Here's how the part is built. I have some questions about the finished solid (model axes, mm). Face numbers are marked on the shaded views. Round coordinates to 2 decimals unless told otherwise and drop trailing zeros. Loops run counter-clockwise (first coordinate to the right, second up) from the corner with the lowest first, then second, coordinate; pieces in that order, holes last. Notation, with made-up numbers: M 62,-38.75 L 70,-38.75 A21 cw 70,-15.75 Z; hole C 55.25,31.25 d11. An arc over 180 degrees is marked long. Answer as a JSON object with one key per item and string values.
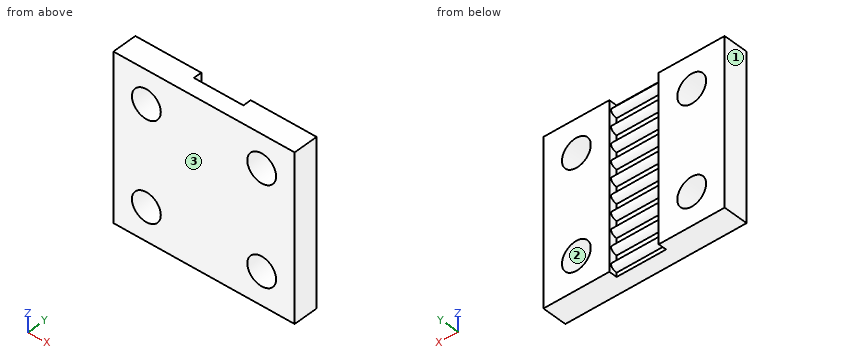
from build123d import *

# Parameters (mm, degrees)
BOSS_EXTRUDE1_DEPTH     = 10
BOSS_EXTRUDE2_START     = -11
SKETCH3_RX              = 0.75
SKETCH3_RY              = 0.5
BOSS_EXTRUDE2_DEPTH     = 14
LPATTERN1_COUNT         = 5
LPATTERN1_PITCH         = 2
LPATTERN1_COL_COUNT     = 6
LPATTERN1_COL_PITCH     = 2
SKETCH4_R               = 1.75
CUT_EXTRUDE2_DEPTH      = 2.0000001
CUT_EXTRUDE2_DEPTH_BACK = 3


with BuildPart() as part:
    # Sketch2 → Boss-Extrude1 (new body, symmetric)
    with BuildSketch(Plane.XY):
        Polygon((-11, 1), (-3, 1), (-3, 0), (3, 0), (3, 1), (11, 1), (11, -2), (-11, -2), align=None)
    extrude(amount=BOSS_EXTRUDE1_DEPTH, both=True)

    # Sketch3 → Boss-Extrude2 (add)
    with BuildSketch(Plane(origin=(0, 0, 0), x_dir=(0, 0, -1), z_dir=(1, 0, 0)).offset(BOSS_EXTRUDE2_START)):
        with Locations(Location((-1, 0), (0, 0, 90))):
            Ellipse(SKETCH3_RX, SKETCH3_RY)
    boss_extrude2 = extrude(amount=BOSS_EXTRUDE2_DEPTH)

    # LPattern1: Boss-Extrude2 ×5
    with Locations(*[(0, 0, i * LPATTERN1_PITCH) for i in range(1, LPATTERN1_COUNT)]):
        add(boss_extrude2)

    # LPattern1 col: Boss-Extrude2 ×6
    with Locations(*[(0, 0, -i * LPATTERN1_COL_PITCH) for i in range(1, LPATTERN1_COL_COUNT)]):
        add(boss_extrude2)

    # Sketch4 → Cut-Extrude2 (cut, two sides)
    with BuildSketch(Plane(origin=(0, 0, 0), x_dir=(1, 0, 0), z_dir=(0, 1, 0))) as cut_extrude2_sk:
        with Locations((-7, 6)):
            Circle(SKETCH4_R)
        with Locations((7, 6)):
            Circle(SKETCH4_R)
        with Locations((7, -6)):
            Circle(SKETCH4_R)
        with Locations((-7, -6)):
            Circle(SKETCH4_R)
    extrude(amount=CUT_EXTRUDE2_DEPTH, mode=Mode.SUBTRACT)
    extrude(cut_extrude2_sk.sketch, amount=-CUT_EXTRUDE2_DEPTH_BACK, mode=Mode.SUBTRACT)


solid = part.part
Item 1: I want a section at B-B on z = -6. List the corners of the cut face in (x, y) for me.
Solution:
{"outline": "M -11,-2 L -8.75,-2 L -8.75,1 L -11,1 Z; M -5.25,-2 L 5.25,-2 L 5.25,1 L 3,1 L 3,0 L -3,0 L -3,1 L -5.25,1 Z; M 8.75,-2 L 11,-2 L 11,1 L 8.75,1 Z"}
Item 2: For P1, Ø0.8, axis at x = -0.5, z = -4, coming from the +Y side; P2, Ø3, axis at x = -7, z = 6, coming from the +Y side, each with a flat end and sliding along its axis, tell me the tip position at first contact or that it passes through.
Solution:
{"P1": "stops at y = 0", "P2": "passes through"}
Item 3: If I drill on L1, parallel to Z at x = 7, y = -1.4; L2, parallel to X at y = -1.1, z = 6; L3, parallel to X at y = 0.1, z = -6, over which ranges is the centre line in solid material (lowest first)? Write a range as from..to.
Solution:
{"L1": "z = -10..-7.75, -4.25..4.25, 7.75..10", "L2": "x = -11..-8.75, -5.25..5.25, 8.75..11", "L3": "x = -11..-8.75, -5.25..-3, 3..5.25, 8.75..11"}
Item 4: We'd pull the mould along X, two halves only. Please class the marked faces 1, 2 and 3: +X half, -X half, draft (parallel to the pull), parting line (faces both ways), or undercut.
Solution:
{"face 1": "-X half", "face 2": "undercut", "face 3": "draft"}
Item 5: I want a section at C-C on y = -0.7. List the corners of the cut face in (x, z) for me.
Solution:
{"outline": "M -11,-10 L 11,-10 L 11,10 L -11,10 Z; hole C -7,-6 d3.5; hole C -7,6 d3.5; hole C 7,-6 d3.5; hole C 7,6 d3.5"}
Item 6: I want a section at A-A on x = -7. List the corners of the cut face in (y, z) for me.
Solution:
{"outline": "M -2,-10 L 1,-10 L 1,-7.75 L -2,-7.75 Z; M -2,-4.25 L 1,-4.25 L 1,4.25 L -2,4.25 Z; M -2,7.75 L 1,7.75 L 1,10 L -2,10 Z"}
Item 7: I want a section at D-D on x = 5.5. List the corners of the cut face in (y, z) for me, plus the area to 3 significant figures.
Solution:
{"outline": "M -2,-10 L 1,-10 L 1,-6.9 L -2,-6.9 Z; M -2,-5.1 L 1,-5.1 L 1,5.1 L -2,5.1 Z; M -2,6.9 L 1,6.9 L 1,10 L -2,10 Z", "area": "49.2 mm2"}
